Geometry check sheet. Reference: the model listing, model coordinates, mm. A direction names the side the tool comes from. Round coordinates to 2 decimals unless told otherwise and drop trailing zeros. Order: outer loops, then holes, each group sorted by start corner. A loop starts at its lowest first (then second) coordinate and runs counter-clockwise, first axis right, second up. Notation, with made-up numbers: (36.25, -10.5) - (45.25, -10.5) arc R25 cw to (45.25, 1.5) - close; hole circle Ø5 at (-40, -25). An arc over 180 degrees is marked (long way). Use a Markdown table: item, result. Add a question column.
(1) Section check C-C on y = -102.5. Record the boundary of the cut face in (x, z).
(2) Thickness scan on line 1 along X through (y, z) = (-217, -556.5); line 2 along Z through (x, y) = (716, -213). Record the ranges inside material, lowest first. Write a range as [from, to].
(3) Section check B-B on z = -650.5. Record the boundary of the cut face in (x, y), then the cut area to 3 significant figures.
(4) Gauge pin test, flat ends, axial feed: P1, Ø1, axis at x = 820.5, z = -48.5, coming from the +Y side; P2, Ø10, axis at x = 393.5, y = -156.5, coming from the -Z side. Record the tip position at first contact, or that the pin passes through.
(5) Access from +Z, -Z, +X, -X, +Y, -Y to the whole of each face (thin tool, end or side, straight path). Record for faces 1 (the face through (795.488, -142, -573)), 2 (the face through (883, 0, -4)).
(6) Section check A-A on x = 22. Record the boundary of the cut face in (y, z).
```python
from build123d import *

# Parameters (mm, degrees)
F0_W     = 600
F0_H     = 800
F0_W_2   = 800
F0_H_2   = 600
F1_DEPTH = 288


with BuildPart() as f1:
    # F0 (on Front) → F1 (new body)
    with BuildSketch(Plane.XZ):
        with Locations((95.488157, 130.783261)):
            Rectangle(F0_W, F0_H)
        with Locations((1195.488157, -569.216739)):
            Rectangle(F0_W_2, F0_H_2)
        Polygon((1595.488157, 530.783261), (395.488157, 530.783261), (395.488157, -269.216739), (795.488157, -269.216739), (1595.488157, -269.216739), align=None)
    extrude(amount=F1_DEPTH)


solid = f1.part
```
Check sheet entries:
| question | item | result |
|---|---|---|
| 1 | outline | (-204.51, -269.22) - (795.49, -269.22) - (795.49, -869.22) - (1595.49, -869.22) - (1595.49, 530.78) - (-204.51, 530.78) - close |
| 2 | line 1 | x = [795.49, 1595.49] |
| 2 | line 2 | z = [-269.22, 530.78] |
| 3 | outline | (795.49, -288) - (1595.49, -288) - (1595.49, 0) - (795.49, 0) - close |
| 3 | area | 230,000 mm2 |
| 4 | P1 | stops at y = 0 |
| 4 | P2 | stops at z = -269.22 |
| 5 | face 1 | -Z, -X, +Y, -Y |
| 5 | face 2 | +Z, -Z, +X, -X, +Y |
| 6 | outline | (-288, -269.22) - (0, -269.22) - (0, 530.78) - (-288, 530.78) - close |
